The model under review builds one solid part; all positions refer to its coordinate system, in mm. Coordinates: 2 decimals unless noted, no trailing zeros. Write each loop counter-clockwise with the first axis right and the second up, starting at its lowest first coordinate (ties: lowest second). Pieces come first, ordered by that corner, then holes. Notation, with made-up numbers: M 9.5,2 L 37.5,2 A16 cw 37.5,14 Z; hole C 14,74.25 d1. An arc over 180 degrees is marked long. Answer as a JSON object with one key per item and string values.
```python
from build123d import *

# Parameters (mm, degrees)
BOSS_EXTRUDE1_DEPTH = 2.5
FILLET1_R           = 0.2
FILLET2_R           = 0.1


with BuildPart() as part:
    # Sketch1 → Boss-Extrude1 (new body)
    with BuildSketch(Plane(origin=(0, 0, 0), x_dir=(1, 0, 0), z_dir=(0, 1, 0))):
        with BuildLine():
            Line((0, 103.6), (0, 105.039339828))
            ThreePointArc((0, 105.039339828), (2.25, 106.1), (0, 107.160660172))
            Line((0, 107.160660172), (0, 108.6))
            ThreePointArc((0, 108.6), (-95.275317005, 52.120763325), (-91.451606784, -58.571013451))
            Line((-91.451606784, -58.571013451), (-90.239544721, -57.794737277))
            ThreePointArc((-90.239544721, -57.794737277), (-90.559855065, -55.32797801), (-88.453189713, -56.650649963))
            Line((-88.453189713, -56.650649963), (-87.24112765, -55.874373789))
            ThreePointArc((-87.24112765, -55.874373789), (-90.888792281, 49.721096506), (0, 103.6))
        make_face()
    extrude(amount=BOSS_EXTRUDE1_DEPTH)

    # Fillet1
    fillet1_edges = [part.edges().sort_by_distance(p)[0] for p in [
        (-88.453189713, 1.25, 56.650649963),
        (-90.239544721, 1.25, 57.794737277),
    ]]
    fillet(fillet1_edges, radius=FILLET1_R)

    # Fillet2
    fillet2_edges = [part.edges().sort_by_distance(p)[0] for p in [
        (0, 1.25, -107.160660172),
        (0, 1.25, -105.039339828),
    ]]
    fillet(fillet2_edges, radius=FILLET2_R)


solid = part.part
```
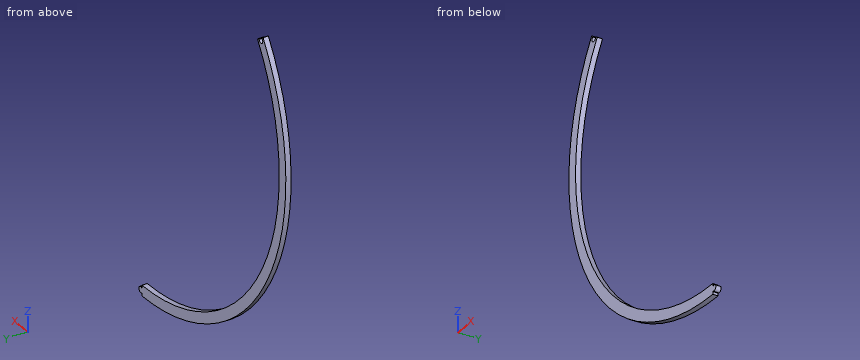
(1) Wall thickness on line 1 along X through (y, z) = (1.2, -38); line 2 along Z through (x, y) = (-62.5, 0.45); line 3 along X through (y, z) = (1.6, 8.5): over which ranges is each line inside the solid? List them lowest first. Write a range as from..to.
Results list:
{"line 1": "-101.73..-96.38", "line 2": "-88.81..-82.62", "line 3": "-108.27..-103.25"}
(2) Add section B-B on z = -10.5. Give the boundary of the cut face in (x, y).
Results list:
{"outline": "M -108.09,0 L -103.07,0 L -103.07,2.5 L -108.09,2.5 Z"}
(3) For pin 1 Ø1.5 at (x, y) = (-25.5, 1) entering from -Z; pin 2 Ø0.6 at (y, z) = (1, -104) entering from +X, all flat-tipped, find the tip position at first contact; note any pin that passes through.
Results list:
{"pin 1": "z = -105.74", "pin 2": "x = 0"}
(4) Add section C-C on x = -53.5. Give the boundary of the cut face in (y, z), and give its area (3 significant figures).
Results list:
{"outline": "M 0,-94.51 L 2.5,-94.51 L 2.5,-88.72 L 0,-88.72 Z", "area": "14.5 mm²"}
(5) Add section A-A on y = 1.85. Give the boundary of the cut face in (x, z) (3 decimals).
Results list:
{"outline": "M -91.452,58.571 A108.6 ccw 0,-108.6 L 0,-107.355 A0.1 cw 0.153,-107.27 A1.375 ccw long 0.153,-104.93 A0.1 cw 0,-104.845 L 0,-103.6 A103.6 cw -87.241,55.874 L -88.148,56.455 A0.2 ccw -88.454,56.312 A1.375 cw long -90.547,57.652 A0.2 ccw -90.545,57.99 Z"}
